Geometry: final body of the model. Coordinates: model frame, mm. A direction names the side the tool comes from. Round coordinates to 2 decimals unless told otherwise and drop trailing zeros. Loops run counter-clockwise (first coordinate to the right, second up) from the corner with the lowest first, then second, coordinate; pieces in that order, holes last. Notation, with made-up numbers: M 84.25,13.25 L 134.25,13.25 A23 ccw 134.25,52.25 Z; hole C -39,63 d5. An arc over 180 degrees is marked long. Answer as a JSON object with one key per item and string values.
```python
from build123d import *

# Parameters (mm, degrees)
SKETCH3_W                                       = 200
SKETCH3_H                                       = 100
BOSS_EXTRUDE2_DEPTH                             = 120
SKETCH4_W                                       = 100
SKETCH4_H                                       = 120
CUT_EXTRUDE1_DEPTH                              = 30
SKETCH5_W                                       = 100
SKETCH5_H                                       = 120
CUT_EXTRUDE2_DEPTH                              = 30
SHELL1_START                                    = 10
SHELL1_OUTLINE_W                                = 100
SHELL1_OUTLINE_H                                = 80
SHELL1_DEPTH                                    = 80
SHELL1_START_2                                  = -90
SHELL1_2_OUTLINE_W                              = 100
SHELL1_2_OUTLINE_H                              = 20
SHELL1_2_DEPTH                                  = 100
CSK_FOR_M2_FLAT_HEAD_MACHINE_SCREW1_D           = 2.4
CSK_FOR_M2_FLAT_HEAD_MACHINE_SCREW1_DEPTH       = 15
CSK_FOR_M2_FLAT_HEAD_MACHINE_SCREW1_CSINK_D     = 4.4
CSK_FOR_M2_FLAT_HEAD_MACHINE_SCREW1_CSINK_ANGLE = 90
CSK_FOR_M2_FLAT_HEAD_MACHINE_SCREW1_TIP         = 0.721032743
CSK_FOR_M2_FLAT_HEAD_MACHINE_SCREW2_D           = 2.4
CSK_FOR_M2_FLAT_HEAD_MACHINE_SCREW2_DEPTH       = 15
CSK_FOR_M2_FLAT_HEAD_MACHINE_SCREW2_CSINK_D     = 4.4
CSK_FOR_M2_FLAT_HEAD_MACHINE_SCREW2_CSINK_ANGLE = 90
CSK_FOR_M2_FLAT_HEAD_MACHINE_SCREW2_TIP         = 0.721032743


# Read off the part's stored shape, not the designer's step: Shell1
with BuildPart() as part:
    # Sketch3 → Boss-Extrude2 (new body)
    with BuildSketch(Plane(origin=(0, 0, 0), x_dir=(1, 0, 0), z_dir=(0, 1, 0))):
        Rectangle(SKETCH3_W, SKETCH3_H)
    extrude(amount=BOSS_EXTRUDE2_DEPTH)

    # Sketch4 → Cut-Extrude1 (cut)
    with BuildSketch(Plane.XY.offset(50)):
        with Locations((-50, 60)):
            Rectangle(SKETCH4_W, SKETCH4_H)
    extrude(amount=-CUT_EXTRUDE1_DEPTH, mode=Mode.SUBTRACT)

    # Sketch5 → Cut-Extrude2 (cut)
    with BuildSketch(Plane(origin=(0, 0, -50), x_dir=(-1, 0, 0), z_dir=(0, 0, -1))):
        with Locations((50, 60)):
            Rectangle(SKETCH5_W, SKETCH5_H)
    extrude(amount=-CUT_EXTRUDE2_DEPTH, mode=Mode.SUBTRACT)

    # Shell1 outline → Shell1 (cut)
    with BuildSketch(Plane.YZ.offset(SHELL1_START)):
        with Locations((60, 0)):
            Rectangle(SHELL1_OUTLINE_W, SHELL1_OUTLINE_H)
    extrude(amount=SHELL1_DEPTH, mode=Mode.SUBTRACT)

    # Shell1 2 outline → Shell1 2 (cut)
    with BuildSketch(Plane.YZ.offset(SHELL1_START_2)):
        with Locations((60, 0)):
            Rectangle(SHELL1_2_OUTLINE_W, SHELL1_2_OUTLINE_H)
    extrude(amount=SHELL1_2_DEPTH, mode=Mode.SUBTRACT)

    # CSK for M2 Flat Head Machine Screw1
    with Locations(Plane.XY.offset(50)):
        with Locations((85, 60), (70, 60), (77.5, 67.5), (77.5, 52.5)):
            CounterSinkHole(CSK_FOR_M2_FLAT_HEAD_MACHINE_SCREW1_D / 2, CSK_FOR_M2_FLAT_HEAD_MACHINE_SCREW1_CSINK_D / 2, depth=CSK_FOR_M2_FLAT_HEAD_MACHINE_SCREW1_DEPTH, counter_sink_angle=CSK_FOR_M2_FLAT_HEAD_MACHINE_SCREW1_CSINK_ANGLE)
            with Locations((0, 0, -(CSK_FOR_M2_FLAT_HEAD_MACHINE_SCREW1_DEPTH + CSK_FOR_M2_FLAT_HEAD_MACHINE_SCREW1_TIP / 2))):  # 118° drill point
                Cone(0, CSK_FOR_M2_FLAT_HEAD_MACHINE_SCREW1_D / 2, CSK_FOR_M2_FLAT_HEAD_MACHINE_SCREW1_TIP, mode=Mode.SUBTRACT)

    # CSK for M2 Flat Head Machine Screw2
    with Locations(Plane.XY.offset(20)):
        with Locations((-85, 60), (-77.179261413, 67.5), (-70, 60), (-77.5, 52.5034295)):
            CounterSinkHole(CSK_FOR_M2_FLAT_HEAD_MACHINE_SCREW2_D / 2, CSK_FOR_M2_FLAT_HEAD_MACHINE_SCREW2_CSINK_D / 2, depth=CSK_FOR_M2_FLAT_HEAD_MACHINE_SCREW2_DEPTH, counter_sink_angle=CSK_FOR_M2_FLAT_HEAD_MACHINE_SCREW2_CSINK_ANGLE)
            with Locations((0, 0, -(CSK_FOR_M2_FLAT_HEAD_MACHINE_SCREW2_DEPTH + CSK_FOR_M2_FLAT_HEAD_MACHINE_SCREW2_TIP / 2))):  # 118° drill point
                Cone(0, CSK_FOR_M2_FLAT_HEAD_MACHINE_SCREW2_D / 2, CSK_FOR_M2_FLAT_HEAD_MACHINE_SCREW2_TIP, mode=Mode.SUBTRACT)


solid = part.part
```
1) Set-up query: faces 1 (the face through (21, 120, -1)), 2 (the face through (0, 59, 35)), 3 (the face through (10, 59, 25)). Return all of +Z, -Z, +X, -X, +Y, -Y with unobstructed straight access to the full face (end or side cutting, diameter ignored); none if empty.
Geometry results:
{"face 1": "+Z, -Z, +X, -X, +Y", "face 2": "+Z, -X, +Y, -Y", "face 3": "none"}
2) Cut plane B-B on y = 14. Return the cut outline in (x, z), and give its area (3 significant figures).
Geometry results:
{"outline": "M -100,-20 L 0,-20 L 0,-50 L 100,-50 L 100,50 L 0,50 L 0,20 L -100,20 Z; hole M -90,-10 L 10,-10 L 10,-40 L 90,-40 L 90,40 L 10,40 L 10,10 L -90,10 Z", "area": "5,600 mm2"}
3) Cut plane A-A on x = -59. Return the cut outline in (y, z), and give its area (3 significant figures).
Geometry results:
{"outline": "M 0,-20 L 120,-20 L 120,20 L 0,20 Z; hole M 10,-10 L 110,-10 L 110,10 L 10,10 Z", "area": "2,800 mm2"}
4) First-contact query: pin 1 (3 mm diameter, centred on x = 77.5, y = 52.5, fed in from +Z); pin 2 (3 mm diameter, centred on x = -77.5, y = 52.5, fed in from +Z); pin 3 (15 mm diameter, centred on y = 55.5, z = 36.5, fed in from -X). Flat tips, straight axial feed; report the tip coordinate or a pass-through.
Geometry results:
{"pin 1": "z = 49.3", "pin 2": "z = 19.3", "pin 3": "x = 0"}
5) Pull-direction query (Y, two-part tool) for faces 4 (the face through (-90, 59, 0)), 5 (the face through (-51, 61, 20)), 6 (the face through (21, 0, -1)); classes: +Y half, -Y half, draft (parallel to the pull), parting line (faces both ways), or undercut.
Geometry results:
{"face 4": "undercut", "face 5": "draft", "face 6": "-Y half"}
6) Line query: probe 1 along Y at (x, z) = (77.5, 42.25); probe 2 along X at (y, z) = (60, 45); probe 3 along Z at (x, y) = (-3, 48). Output: solid intervals per line, ascending.
Geometry results:
{"probe 1": "0 to 51.3, 53.7 to 66.3, 68.7 to 120", "probe 2": "0 to 68.8, 71.2 to 83.8, 86.2 to 100", "probe 3": "-20 to -10, 10 to 20"}
